The listing builds one solid part. Answer for the finished solid, in the listing's coordinates (mm). A direction names the side the tool comes from. Round coordinates to 2 decimals unless told otherwise and drop trailing zeros. Write each loop counter-clockwise with the first axis right and the second up, starting at its lowest first coordinate (ties: lowest second). Pieces come first, ordered by that corner, then holes. Notation, with made-up numbers: (-22, 34.5) - (13, 34.5) arc R17 cw to (13, 64.5) - close; hole circle Ø4 at (49, -40). An arc over 180 degrees is marked (long way). Return JSON: item names as keys, results as strings. Group by question number.
(1) Section C-C, the plane y = 20 is taken. Write down the section's boundary in (x, z), then the cut area to 3 significant figures.
(2) Each of these flat-tipped pins is pushed along its axis until it touches: pin 1 (5 mm diameter, centred on x = -8.5, z = 5.5, fed in from -Y); pin 2 (3.5 mm diameter, centred on x = -21, y = 0, fed in from -Z); pin 3 (7 mm diameter, centred on x = 0, y = 21, fed in from +Z); pin 4 (2 mm diameter, centred on y = 6.5, z = 31.5, fed in from +X) (3 decimals). Where does it stop, or does it pass through?
(3) Find the intervals of material crossed by line 1 along Y through (x, z) = (0, 3.5); line 2 along Y through (x, z) = (-2.5, 5.5); line 3 along Z through (x, y) = (-13, -19), in increasing order. Write a range as [from, to].
(4) Which of the six approach directions +Z, -Z, +X, -X, +Y, -Y give full straight-line access (tool end or side, diameter ignored) to faces 4 (the cylindrical face through (-18.07, 0.65, 6.48)), 5 (the flat face through (12, -12, 8)), 6 (the cylindrical face through (24.794, 2.419, 2.465))?
(5) Section A-A, the plane y = 0 is taken. Write down the section's boundary in (x, z).
(6) Section D-D, the plane z = 36.5 is taken. Write down the section's boundary in (x, y).
(7) Determine the mould class of faces 1 (the flat face through (-0.2, -10.4, 42)), 2 (the cylindrical face through (-3.47, 15.62, 24.76)), 3 (the cylindrical face through (-2.17, 9.76, 20.71)) for opening direction X: +X half, -X half, draft (parallel to the pull), parting line (faces both ways), or undercut.
Autodesk Inventor part; units mm, degrees
ref_plane "YZ Plane" through (0, 0, 0) normal (1, 0, 0) x (0, 1, 0)
ref_plane "XZ Plane" through (0, 0, 0) normal (0, 1, 0) x (-1, 0, 0)
ref_plane "XY Plane" through (0, 0, 0) normal (0, 0, 1) x (1, 0, 0)
sketch "Sketch1" plane through (0, 0, 0) normal (0, 0, 1) x (1, 0, 0)
  circle A0 centre (0, 0) radius 27
  circle A1 centre (0, 0) radius 10
  dimension "d0" = 54
  dimension "d1" = 20
extrude "Extrusion1" add sketch "Sketch1" along normal blind 8
sketch "Sketch2" plane through (0, 0, 8) normal (0, 0, 1) x (1, 0, 0)
  circle A0 centre (0, 0) radius 10
  circle A1 centre (0, 0) radius 16
  dimension "d4" = 32
extrude "Extrusion2" add sketch "Sketch2" along normal blind 34
sketch "Sketch3" plane through (0, 0, 0) normal (0, 0, -1) x (-1, 0, 0)
  circle A0 centre (0, 0) radius 21 construction
  circle A1 centre (0, 21) radius 4.5
  dimension "d7" = 42
  dimension "d8" = 9
extrude "Extrusion3" cut sketch "Sketch3" against normal blind 5
sketch "Sketch4" plane through (0, 21, 5) normal (0, 0, -1) x (-1, 0, 0)
  circle A0 centre (0, 0) radius 4.5
  circle A1 centre (0, 0) radius 3
  point P0 (0, -21)
  dimension "d11" = 6
extrude "Extrusion4" cut sketch "Sketch4" against normal through all contours A1
pattern_circular "Circular Pattern1" count 4 over 360 about axis through (0, 0, 0) along (0, 0, 1) of "Extrusion4", "Extrusion3"
properties part number "LMF20UU" material "Aluminum 6061"
Working result:
{
 "1": {"outline": "(-18.14, 0) - (-4.39, 0) - (-4.39, 5) - (-2.83, 5) - (-2.83, 8) - (-18.14, 8) - close; (2.83, 5) - (4.39, 5) - (4.39, 0) - (18.14, 0) - (18.14, 8) - (2.83, 8) - close", "area": "229 mm^2"},
 "2": {"pin 1": "stops at y = -26.32", "pin 2": "passes through", "pin 3": "stops at z = 8", "pin 4": "stops at x = 15.025"},
 "3": {"line 1": "y = [-27, -25.5], [-16.5, -10], [10, 16.5], [25.5, 27]", "line 2": "y = [-26.88, -22.66], [-19.34, -9.68], [9.68, 19.34], [22.66, 26.88]", "line 3": "z = [0, 8]"},
 "4": {"face 4": "+Z, -Z", "face 5": "+Z", "face 6": "-Z"},
 "5": {"outline": "(-27, 0) - (-25.5, 0) - (-25.5, 5) - (-24, 5) - (-24, 8) - (-27, 8) - close; (-18, 5) - (-16.5, 5) - (-16.5, 0) - (-10, 0) - (-10, 42) - (-16, 42) - (-16, 8) - (-18, 8) - close; (10, 0) - (16.5, 0) - (16.5, 5) - (18, 5) - (18, 8) - (16, 8) - (16, 42) - (10, 42) - close; (24, 5) - (25.5, 5) - (25.5, 0) - (27, 0) - (27, 8) - (24, 8) - close"},
 "6": {"outline": "circle Ø32 at (0, 0); hole circle Ø20 at (0, 0)"},
 "7": {"face 1": "draft", "face 2": "parting line", "face 3": "undercut"}
}
